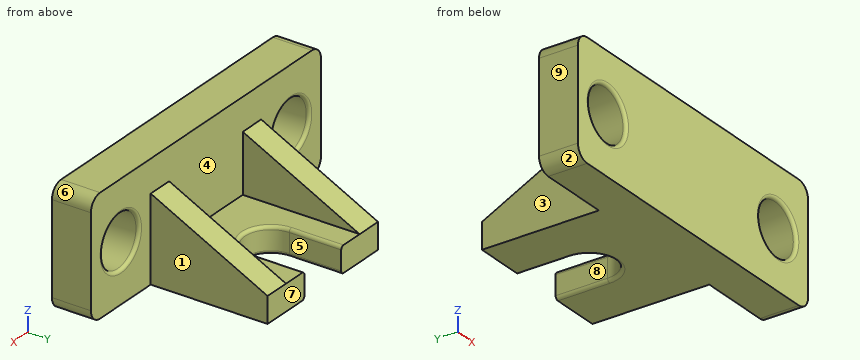
from build123d import *

# Parameters (mm, degrees)
SKETCH1_W           = 100
SKETCH1_H           = 12
BOSS_EXTRUDE1_DEPTH = 36
SKETCH2_W           = 48
SKETCH2_H           = 26
BOSS_EXTRUDE2_DEPTH = 36
SKETCH3_W           = 32
SKETCH3_H           = 18
CUT_EXTRUDE1_DEPTH  = 36
CUT_EXTRUDE2_START  = -48
CUT_EXTRUDE2_DEPTH  = 48
CUT_EXTRUDE5_DEPTH  = 36
SKETCH6_R           = 8
CUT_EXTRUDE6_DEPTH  = 36
FILLET1_R           = 4
FILLET2_R           = 1


with BuildPart() as part:
    # Sketch1 → Boss-Extrude1 (new body)
    with BuildSketch(Plane.XY):
        with Locations((50, 6)):
            Rectangle(SKETCH1_W, SKETCH1_H)
    extrude(amount=-BOSS_EXTRUDE1_DEPTH)

    # Sketch2 → Boss-Extrude2 (add)
    with BuildSketch(Plane(origin=(0, 12, 0), x_dir=(1, 0, 0), z_dir=(0, 1, 0))):
        with Locations((50, 23)):
            Rectangle(SKETCH2_W, SKETCH2_H)
    extrude(amount=BOSS_EXTRUDE2_DEPTH)

    # Sketch3 → Cut-Extrude1 (cut)
    with BuildSketch(Plane(origin=(0, 48, 0), x_dir=(1, 0, 0), z_dir=(0, 1, 0))):
        with Locations((50, 19)):
            Rectangle(SKETCH3_W, SKETCH3_H)
    extrude(amount=-CUT_EXTRUDE1_DEPTH, mode=Mode.SUBTRACT)

    # Sketch4 → Cut-Extrude2 (cut)
    with BuildSketch(Plane.ZY.offset(-26).offset(CUT_EXTRUDE2_START)):
        Polygon((-28, 48), (-10, 12), (-10, 48), align=None)
    extrude(amount=CUT_EXTRUDE2_DEPTH, mode=Mode.SUBTRACT)

    # Sketch5 → Cut-Extrude5 (cut)
    with BuildSketch(Plane.XY.offset(-28)):
        with BuildLine():
            Line((42, 48), (58, 48))
            Line((58, 48), (58, 32))
            ThreePointArc((58, 32), (50, 24), (42, 32))
            Line((42, 32), (42, 48))
        make_face()
    extrude(amount=-CUT_EXTRUDE5_DEPTH, mode=Mode.SUBTRACT)

    # Sketch6 → Cut-Extrude6 (cut)
    with BuildSketch(Plane(origin=(0, 12, 0), x_dir=(1, 0, 0), z_dir=(0, 1, 0))):
        with Locations((13, 18)):
            Circle(SKETCH6_R)
        with Locations((87, 18)):
            Circle(SKETCH6_R)
    extrude(amount=-CUT_EXTRUDE6_DEPTH, mode=Mode.SUBTRACT)

    # Fillet1
    fillet1_edges = [part.edges().sort_by_distance(p)[0] for p in [
        (100, 6, -36),
        (0, 6, -36),
        (100, 6, 0),
        (0, 6, 0),
    ]]
    fillet(fillet1_edges, radius=FILLET1_R)

    # Fillet2
    fillet2_edges = [part.edges().sort_by_distance(p)[0] for p in [
        (50, 24, -36),
        (42, 40, -36),
        (58, 40, -36),
        (50, 24, -28),
        (58, 40, -28),
        (42, 40, -28),
        (79, 0, -18),
        (79, 12, -18),
        (5, 0, -18),
        (5, 12, -18),
    ]]
    fillet(fillet2_edges, radius=FILLET2_R)


solid = part.part
Verification items for the finished model (mm, model axes). Face numbers are marked on the shaded views. A direction names the side the tool comes from. Round coordinates to 2 decimals unless told otherwise and drop trailing zeros. Loops run counter-clockwise (first coordinate to the right, second up) from the corner with the lowest first, then second, coordinate; pieces in that order, holes last. Notation, with made-up numbers: (38, 45) - (92, 45) arc R19 ccw to (92, 56) - close; hole circle Ø3 at (-11, 58.25). An arc over 180 degrees is marked (long way). Use a Markdown table: item, result. Add a question column.
1. Section check A-A, the plane y = 36. Record the boundary of the cut face in (x, z).
2. Access from +Z, -Z, +X, -X, +Y, -Y to the whole of each face (thin tool, end or side, straight path). Record for the marked faces 1, 2, 3, 4 and 5.
3. Section check C-C, the plane z = -18. Record the boundary of the cut face in (x, y), plus the area to 3 significant figures.
4. Gauge pin test, flat ends, axial feed: pin 1 (3 mm diameter, centred on y = 43.5, z = -30.5, fed in from -X); pin 2 (1.5 mm diameter, centred on y = 18.5, z = -19, fed in from +X); pin 3 (10 mm diameter, centred on x = 68, y = 22, fed in from +Z). Record the tip position at first contact, or that the pin passes through.
5. Thickness scan on probe 1 along X at (y, z) = (3, -18); probe 2 along Z at (x, y) = (87, 3.75); probe 3 along X at (y, z) = (2, -14). Record the ranges inside material, lowest first. Write a range as [from, to].
6. Release check for a two-part mould opening along X. For the marked faces 6, 7, 8 and 9 record: released by +X, released by -X, zero draft, split by the parting line, or undercut.
7. Section check D-D, the plane y = 45. Record the boundary of the cut face in (x, z).
8. Section check B-B, the plane x = 87. Record the boundary of the cut face in (y, z), plus the area to 3 significant figures.
Checks:
| question | item | result |
|---|---|---|
| 1 | outline | (26, -36) - (41, -36) arc R1 ccw to (42, -35) - (42, -29) arc R1 ccw to (41, -28) - (34, -28) - (34, -22) - (26, -22) - close; (58, -35) arc R1 ccw to (59, -36) - (74, -36) - (74, -22) - (66, -22) - (66, -28) - (59, -28) arc R1 ccw to (58, -29) - close |
| 2 | face 1 | +Z, -Z, +X, +Y |
| 2 | face 2 | -Z, -X, +Y, -Y |
| 2 | face 3 | +Z, -Z, -X, +Y |
| 2 | face 4 | +Z, +Y |
| 2 | face 5 | +Z, -Z, +Y |
| 3 | outline | (0, 0) - (4, 0) arc R1 ccw to (5, 1) - (5, 11) arc R1 ccw to (4, 12) - (0, 12) - close; (21, 1) arc R1 ccw to (22, 0) - (78, 0) arc R1 ccw to (79, 1) - (79, 11) arc R1 ccw to (78, 12) - (74, 12) - (74, 28) - (66, 28) - (66, 12) - (34, 12) - (34, 28) - (26, 28) - (26, 12) - (22, 12) arc R1 ccw to (21, 11) - close; (95, 1) arc R1 ccw to (96, 0) - (100, 0) - (100, 12) - (96, 12) arc R1 ccw to (95, 11) - close |
| 3 | area | 1,070 mm^2 |
| 4 | pin 1 | stops at x = 26 |
| 4 | pin 2 | stops at x = 74 |
| 4 | pin 3 | stops at z = -12.5 |
| 5 | probe 1 | x = [0, 5], [21, 79], [95, 100] |
| 5 | probe 2 | z = [-36, -26], [-10, 0] |
| 5 | probe 3 | x = [0, 6.07], [19.93, 80.07], [93.93, 100] |
| 6 | face 6 | released by +X |
| 6 | face 7 | zero draft |
| 6 | face 8 | undercut |
| 6 | face 9 | released by -X |
| 7 | outline | (26, -36) - (41, -36) arc R1 ccw to (42, -35) - (42, -29) arc R1 ccw to (41, -28) - (34, -28) - (34, -26.5) - (26, -26.5) - close; (58, -35) arc R1 ccw to (59, -36) - (74, -36) - (74, -26.5) - (66, -26.5) - (66, -28) - (59, -28) arc R1 ccw to (58, -29) - close |
| 8 | outline | (0, -36) - (12, -36) - (12, -27) arc R1 ccw to (11, -26) - (1, -26) arc R1 ccw to (0, -27) - close; (0, -9) arc R1 ccw to (1, -10) - (11, -10) arc R1 ccw to (12, -9) - (12, 0) - (0, 0) - close |
| 8 | area | 239 mm^2 |
